Part print with two shaded views. Sizes in mm from the minimum x, y, z corner. Give positions to 0.01 mm unless a question says otherwise; leave off trailing zeros. Order: outer loops, then holes, each group sorted by start corner. A loop starts at its lowest first (then second) coordinate and runs counter-clockwise, first axis right, second up. Notation, with made-up numbers: (79, -14) -> (95, -14) arc R12 cw to (95, 9) -> close; hole circle Ø5 at (85.25, -16.5). An arc over 180 degrees is marked (long way). Answer as CSV lines item,"result".
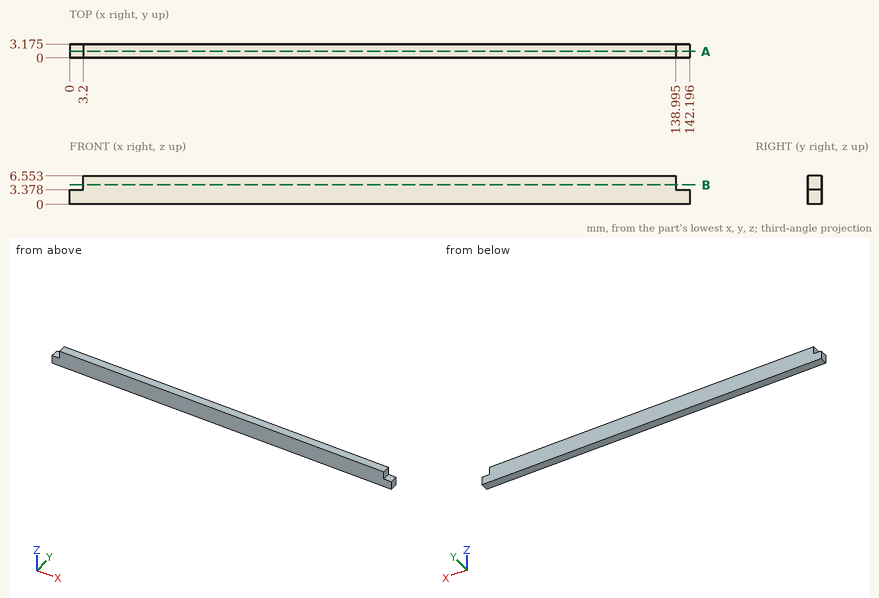
1) Band-saw the part on A-A, the plane y = 1.5. Write the cut outline in (x, z) (1 decimal).
Data:
outline,"(0, 0) -> (142.2, 0) -> (142.2, 3.4) -> (139, 3.4) -> (139, 6.6) -> (3.2, 6.6) -> (3.2, 3.4) -> (0, 3.4) -> close"
2) Pin check, flat tips, straight feed: P1, Ø1, axis at y = 1.5, z = 4, coming from the -X side; P2, Ø1.6, axis at x = 141, y = 1.5, coming from the +Z side. Stop position of each tip, or through.
Data:
P1,"stops at x = 3.2"
P2,"stops at z = 3.38"
3) Wall check: line 1 along X through (y, z) = (0.2, 3.75) (1 decimal). Give the ranges that are in metal, low to high. Write a range as [from, to].
Data:
line 1,"x = [3.2, 139]"
4) Band-saw the part on B-B, the plane z = 4.5. Write the cut outline in (x, y) (1 decimal).
Data:
outline,"(3.2, 0) -> (139, 0) -> (139, 3.2) -> (3.2, 3.2) -> close"
